Can you work these out from the model? Positions are in its coordinate system, mm. Round coordinates to 2 decimals unless told otherwise and drop trailing zeros. Loops run counter-clockwise (first coordinate to the right, second up) from the corner with the lowest first, then second, coordinate; pieces in that order, holes last. Notation, with made-up numbers: (79.25, 69) -> (108.25, 69) arc R13 ccw to (108.25, 86) -> close; hole circle Ø1 at (17.5, 16). An arc over 180 degrees is marked (long way). Use a Markdown table: item, result.
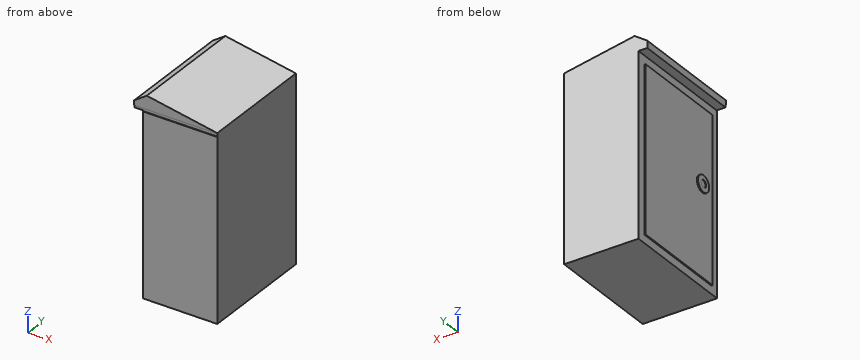
from build123d import *

# Parameters (mm, degrees)
PAD022_DEPTH    = 1000
SKETCH031_W     = 855.878418
SKETCH031_H     = 26.746094
POCKET007_DEPTH = 5
SKETCH033_W     = 1407.922851
SKETCH033_H     = 855.013962
PAD024_DEPTH    = 10
SKETCH034_R     = 70.506238
PAD025_DEPTH    = 10
SKETCH035_R     = 31.935014
POCKET008_DEPTH = 5


with BuildPart() as part:
    # Sketch029 → Pad022 (new body)
    with BuildSketch(Plane.XZ):
        Polygon((-2829.030029, 2082.267822), (-2829.030029, 529.913818), (-2191.9729, 529.913818), (-2191.9729, 2108.837402), (-2796.181885, 2217.138916), (-2904.483643, 2143.037842), (-2904.483643, 2082.267822), align=None)
    extrude(amount=PAD022_DEPTH)

    # Sketch031 (on Face9 of Pad022) → Pocket007 (cut)
    with BuildSketch(Plane.XZ.offset(1000)):
        with Locations((-2559.213379, 2089.656738)):
            Rectangle(SKETCH031_W, SKETCH031_H)
    extrude(amount=-POCKET007_DEPTH, mode=Mode.SUBTRACT)

    # Sketch033 (on Face1 of Pocket007) → Pad024 (join)
    with BuildSketch(Plane(origin=(-2829.030029, 0, 0), x_dir=(0, 0, -1), z_dir=(-1, 0, 0))):
        with Locations((-1303.355225, 502.411583)):
            Rectangle(SKETCH033_W, SKETCH033_H)
    extrude(amount=PAD024_DEPTH)

    # Sketch034 (on Face17 of Pad024) → Pad025 (join)
    with BuildSketch(Plane(origin=(-2839.030029, 0, 0), x_dir=(0, 0, -1), z_dir=(-1, 0, 0))):
        with Locations((-1372.109253, 798.877693)):
            Circle(SKETCH034_R)
    extrude(amount=PAD025_DEPTH)

    # Sketch035 (on Face20 of Pad025) → Pocket008 (cut)
    with BuildSketch(Plane(origin=(-2849.030029, 0, 0), x_dir=(0, 0, -1), z_dir=(-1, 0, 0))):
        with Locations((-1372.115967, 799.249336)):
            Circle(SKETCH035_R)
    extrude(amount=-POCKET008_DEPTH, mode=Mode.SUBTRACT)


with BuildPart() as part_1:
    # Body018 placement: moved
    add(part.part.moved(Location((0, 747, 0))))


solid = part_1.part
1. I want a section at A-A (z = 1515). Please give me the cut outline in (x, y).
Answer sheet:
| item | result |
|---|---|
| outline | (-2839.03, -182.92) -> (-2829.03, -182.92) -> (-2829.03, -253) -> (-2191.97, -253) -> (-2191.97, 747) -> (-2829.03, 747) -> (-2829.03, 672.1) -> (-2839.03, 672.1) -> close |
2. Will these pins go through, and if not, where does the flat tip stop? pin 1 Ø1 at (x, y) = (-2611.5, 147) entering from +Z; pin 2 Ø8 at (x, y) = (-2835, 38) entering from -Z; pin 3 Ø10 at (y, z) = (465.5, 1750.5) entering from -X.
Answer sheet:
| item | result |
|---|---|
| pin 1 | stops at z = 2184.13 |
| pin 2 | stops at z = 599.39 |
| pin 3 | stops at x = -2839.03 |
3. I need wall thicknesses on line 1 (Z direction, x = -2382.5, y = 665); line 2 (X direction, y = 289.5, z = 2043.5); line 3 (X direction, y = 92, z = 982). Which ranges of each line are inside material? Lowest first, please.
Answer sheet:
| item | result |
|---|---|
| line 1 | z = 529.91 to 2142.99 |
| line 2 | x = -2829.03 to -2191.97 |
| line 3 | x = -2839.03 to -2191.97 |
4. I want a section at C-C (y = 259). Please give me the cut outline in (x, z).
Answer sheet:
| item | result |
|---|---|
| outline | (-2904.48, 2082.27) -> (-2829.03, 2082.27) -> (-2829.03, 2007.32) -> (-2839.03, 2007.32) -> (-2839.03, 599.39) -> (-2829.03, 599.39) -> (-2829.03, 529.91) -> (-2191.97, 529.91) -> (-2191.97, 2108.84) -> (-2796.18, 2217.14) -> (-2904.48, 2143.04) -> close |
5. I want a section at B-B (x = -2454). Please give me the cut outline in (y, z).
Answer sheet:
| item | result |
|---|---|
| outline | (-253, 529.91) -> (747, 529.91) -> (747, 2155.8) -> (-253, 2155.8) -> (-253, 2103.03) -> (-248, 2103.03) -> (-248, 2076.28) -> (-253, 2076.28) -> close |
